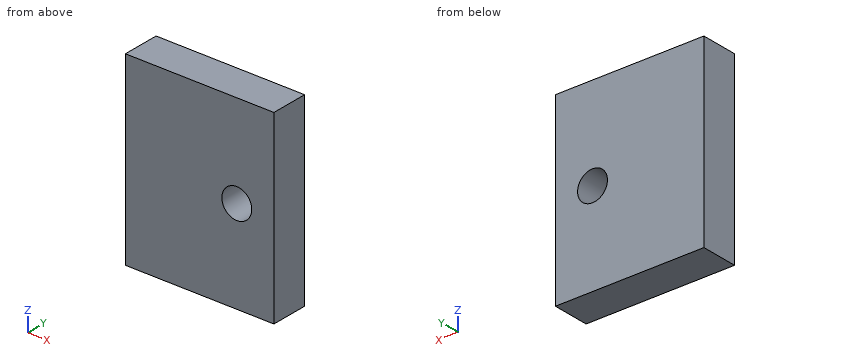
from build123d import *

# Parameters (mm, degrees)
SKETCH2_W                   = 25.4
SKETCH2_H                   = 31.75
BOSS_EXTRUDE1_DEPTH         = 6.35
F_1_4_20_TAPPED_HOLE1_D     = 5.1054
F_1_4_20_TAPPED_HOLE1_DEPTH = 19.05
F_1_4_20_TAPPED_HOLE1_TIP   = 1.533816902


with BuildPart() as part:
    # Sketch2 → Boss-Extrude1 (new body)
    with BuildSketch(Plane(origin=(0, 0, 0), x_dir=(1, 0, 0), z_dir=(0, 1, 0))):
        with Locations((12.7, 15.875)):
            Rectangle(SKETCH2_W, SKETCH2_H)
    extrude(amount=BOSS_EXTRUDE1_DEPTH)

    # 1/4-20 Tapped Hole1
    with Locations(Plane(origin=(19.05, 6.35, -15.875), x_dir=(0, 0, 1), z_dir=(0, 1, 0))):
        with Locations((0, 0)):
            Hole(F_1_4_20_TAPPED_HOLE1_D / 2, depth=F_1_4_20_TAPPED_HOLE1_DEPTH)
            with Locations((0, 0, -(F_1_4_20_TAPPED_HOLE1_DEPTH + F_1_4_20_TAPPED_HOLE1_TIP / 2))):  # 118° drill point
                Cone(0, F_1_4_20_TAPPED_HOLE1_D / 2, F_1_4_20_TAPPED_HOLE1_TIP, mode=Mode.SUBTRACT)


solid = part.part
Geometry check sheet. Reference: the model listing, model coordinates, mm. Coordinates: 2 decimals unless noted, no trailing zeros. Order: outer loops, then holes, each group sorted by start corner. A loop starts at its lowest first (then second) coordinate and runs counter-clockwise, first axis right, second up. Notation, with made-up numbers: (85.25, 12) -> (117.25, 12) arc R26 ccw to (117.25, 45) -> close; hole circle Ø11 at (40, 87.5). An arc over 180 degrees is marked (long way). Use a Markdown table: item, result. Add a question column.
1. Cross-section at A-A (x = 19.05). Enter the section's corners in (y, z).
2. Cross-section at B-B (y = 2.5). Enter the section's corners in (x, z) (3 decimals), and give its area (3 significant figures).
3. Material ranges on L1, parallel to X at y = 4.5, z = -16; L2, parallel to X at y = 5.25, z = -18; L3, parallel to Z at x = 17, y = 3.75, recorded low to high.
4. Go/stop test with a flat-tipped pin: pin 1 Ø3 at (x, z) = (19.05, -15.875) entering from -Y. Record where the tip stops, or that it passes through.
Filled sheet:
| question | item | result |
|---|---|---|
| 1 | outline | (0, -31.75) -> (6.35, -31.75) -> (6.35, -18.43) -> (0, -18.43) -> close; (0, -13.32) -> (6.35, -13.32) -> (6.35, 0) -> (0, 0) -> close |
| 2 | outline | (0, -31.75) -> (25.4, -31.75) -> (25.4, 0) -> (0, 0) -> close; hole circle Ø5.105 at (19.05, -15.875) |
| 2 | area | 786 mm2 |
| 3 | L1 | 0 to 16.5, 21.6 to 25.4 |
| 3 | L2 | 0 to 17.64, 20.46 to 25.4 |
| 3 | L3 | -31.75 to -17.4, -14.35 to 0 |
| 4 | pin 1 | through |
